The figure shows three views and two pictorial views of one solid part (mm, origin at its lowest corner). Answer the questions. A direction names the side the tool comes from. Round coordinates to 2 decimals unless told otherwise and drop trailing zeros. Order: outer loops, then holes, each group sorted by start corner. A loop starts at its lowest first (then second) coordinate and runs counter-clockwise, first axis right, second up. Notation, with made-up numbers: (83, 77.25) - (107, 77.25) arc R21 ccw to (107, 96.25) - close; hole circle Ø5 at (22.25, 45.25). An arc over 180 degrees is marked (long way). One line per item, written item: value. Start each with the question number.
1. Section C-C, the plane x = 12.4 is taken. Give the vertices of the cut face in (y, z), then the cut area to 3 significant figures.
2. Straight lines are drawn through the part: line 1 (Y direction, x = 12.4, z = 0.35); line 2 (X direction, y = 6, z = 2.75); line 3 (X direction, y = 13.1, z = 0.35). For each, find the intervals that lie inside material, in ascending order.
3. Section D-D, the plane x = 20.25 is taken. Give the vertices of the cut face in (y, z), then the cut area to 3 significant figures.
4. Section B-B, the plane y = 1.7 is taken. Give the vertices of the cut face in (x, z), then the cut area to 3 significant figures.
5. A tool of negligible diameter and unlimited length cuts with its end or side. For the marked faces 1, 2, 3, 4 and 5, from which of +Z, -Z, +X, -X, +Y, -Y can it reach the whole face along a straight path? Write none if from no direction.
6. Flat-ended cylindrical pins translate along their axes: P1, Ø3, axis at y = 10.5, z = 6.5, coming from the +X side; P2, Ø3, axis at x = 10, y = 12.5, coming from the -Z side; P3, Ø2, axis at x = 12.4, y = 13.1, coming from the +Z side; P4, Ø2, axis at x = 2.5, z = 8.5, coming from the +Y side. Find the tip coordinate at first contact, or state that the pin passes through.
7. For a pull along X with two mould halves and no side action, classify the marked faces 6, 7 and 8 as released by +X, released by -X, zero draft, split by the parting line, or undercut.
8. Section A-A, the plane z = 8 is taken. Give the vertices of the cut face in (x, y), then the cut area to 3 significant figures.
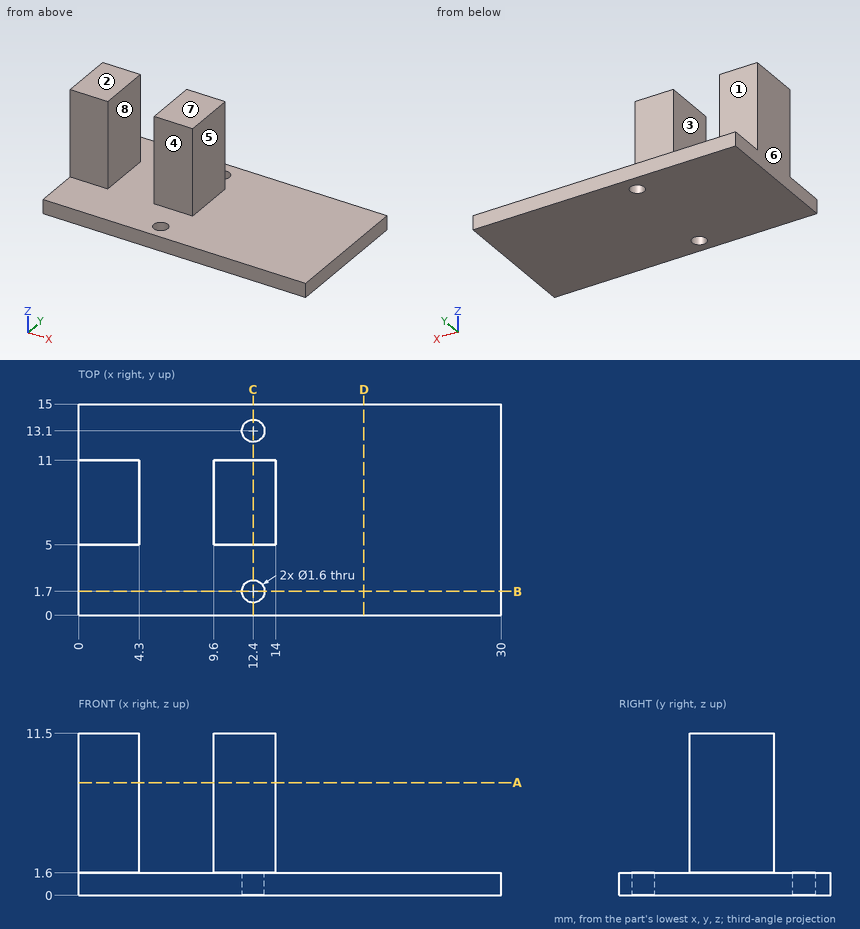
Answer list:
1. outline: (0, 0) - (0.9, 0) - (0.9, 1.6) - (0, 1.6) - close; (2.5, 0) - (12.3, 0) - (12.3, 1.6) - (11, 1.6) - (11, 11.5) - (5, 11.5) - (5, 1.6) - (2.5, 1.6) - close; (13.9, 0) - (15, 0) - (15, 1.6) - (13.9, 1.6) - close
1. area: 78.3 mm²
2. line 1: y = 0 to 0.9, 2.5 to 12.3, 13.9 to 15
2. line 2: x = 0 to 4.3, 9.6 to 14
2. line 3: x = 0 to 11.6, 13.2 to 30
3. outline: (0, 0) - (15, 0) - (15, 1.6) - (0, 1.6) - close
3. area: 24.0 mm²
4. outline: (0, 0) - (11.6, 0) - (11.6, 1.6) - (0, 1.6) - close; (13.2, 0) - (30, 0) - (30, 1.6) - (13.2, 1.6) - close
4. area: 45.4 mm²
5. face 1: +Z, +X, -X, +Y
5. face 2: +Z, +X, -X, +Y, -Y
5. face 3: +Z, +Y, -Y
5. face 4: +Z, +X, -X, -Y
5. face 5: +Z, +X, +Y, -Y
6. P1: stops at x = 14
6. P2: stops at z = 0
6. P3: stops at z = 1.6
6. P4: stops at y = 11
7. face 6: released by -X
7. face 7: zero draft
7. face 8: undercut
8. outline: (0, 5) - (4.3, 5) - (4.3, 11) - (0, 11) - close; (9.6, 5) - (14, 5) - (14, 11) - (9.6, 11) - close
8. area: 52.2 mm²
